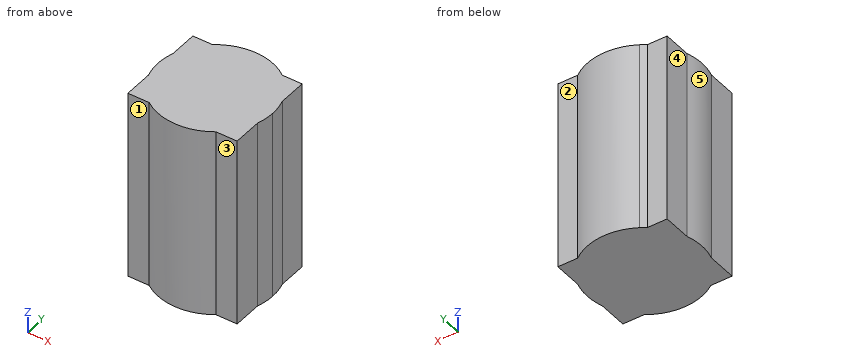
```python
from build123d import *

# Parameters (mm, degrees)
F1_DEPTH = 50.8


with BuildPart() as f1:
    # F0 (on Top) → F1 (new body)
    with BuildSketch(Plane.XY):
        with BuildLine():
            ThreePointArc((14.5472735167, -4.6368075466), (15.087019572, -2.3462718145), (15.2683709345, 0))
            ThreePointArc((15.2683709345, 0), (15.087019572, 2.3462718145), (14.5472735167, 4.6368075466))
            Line((14.5472735167, 4.6368075466), (14.5472735167, -4.6368075466))
        make_face()
        with BuildLine():
            Line((14.5472735167, -4.6368075466), (14.5472735167, 4.6368075466))
            ThreePointArc((14.5472735167, 4.6368075466), (12.4889100158, 8.783523075), (9.2823821573, 12.1227279305))
            Line((9.2823821573, 12.1227279305), (0, 12.1227279305))
            Line((0, 12.1227279305), (-7.8358159836, 12.1227279305))
            Line((-7.8358159836, 12.1227279305), (-9.2823821573, 12.1227279305))
            ThreePointArc((-9.2823821573, 12.1227279305), (-12.4889108979, 8.7835218208), (-14.547274448, 4.6368046247))
            Line((-14.547274448, 4.6368046247), (-14.547274448, -4.6368046247))
            ThreePointArc((-14.547274448, -4.6368046247), (-12.3495786547, -8.9783661121), (-8.8974988368, -12.4079678208))
            Line((-8.8974988368, -12.4079678208), (8.8974988368, -12.4079678208))
            ThreePointArc((8.8974988368, -12.4079678208), (12.349577753, -8.9783673524), (14.5472735167, -4.6368075466))
        make_face()
        with BuildLine():
            ThreePointArc((9.2823821573, 12.1227279305), (12.4889100158, 8.783523075), (14.5472735167, 4.6368075466))
            Line((14.5472735167, 4.6368075466), (14.5472735167, 12.1227279305))
            Line((14.5472735167, 12.1227279305), (9.2823821573, 12.1227279305))
        make_face()
        with BuildLine():
            Line((14.5472735167, -12.4079678208), (14.5472735167, -4.6368075466))
            ThreePointArc((14.5472735167, -4.6368075466), (12.349577753, -8.9783673524), (8.8974988368, -12.4079678208))
            Line((8.8974988368, -12.4079678208), (14.5472735167, -12.4079678208))
        make_face()
        with BuildLine():
            Line((0, 12.1227279305), (9.2823821573, 12.1227279305))
            ThreePointArc((9.2823821573, 12.1227279305), (0.8740812186, 15.2433307717), (-7.8358159836, 13.1043175658))
            Line((-7.8358159836, 13.1043175658), (-7.8358159836, 12.1227279305))
            Line((-7.8358159836, 12.1227279305), (0, 12.1227279305))
        make_face()
        with BuildLine():
            ThreePointArc((-8.8974988368, -12.4079678208), (0, -15.2683709345), (8.8974988368, -12.4079678208))
            Line((8.8974988368, -12.4079678208), (-8.8974988368, -12.4079678208))
        make_face()
        with BuildLine():
            Line((-7.8358159836, 12.1227279305), (-7.8358159836, 13.1043175658))
            ThreePointArc((-7.8358159836, 13.1043175658), (-8.5731590707, 12.6342429351), (-9.2823821573, 12.1227279305))
            Line((-9.2823821573, 12.1227279305), (-7.8358159836, 12.1227279305))
        make_face()
        with BuildLine():
            Line((-14.547274448, -12.4079678208), (-8.8974988368, -12.4079678208))
            ThreePointArc((-8.8974988368, -12.4079678208), (-12.3495786547, -8.9783661121), (-14.547274448, -4.6368046247))
            Line((-14.547274448, -4.6368046247), (-14.547274448, -12.4079678208))
        make_face()
        with BuildLine():
            ThreePointArc((-14.547274448, 4.6368046247), (-12.4889108979, 8.7835218208), (-9.2823821573, 12.1227279305))
            Line((-9.2823821573, 12.1227279305), (-14.547274448, 12.1227279305))
            Line((-14.547274448, 12.1227279305), (-14.547274448, 4.6368046247))
        make_face()
        with BuildLine():
            ThreePointArc((-14.547274448, 4.6368046247), (-15.2683709345, 0), (-14.547274448, -4.6368046247))
            Line((-14.547274448, -4.6368046247), (-14.547274448, 4.6368046247))
        make_face()
    extrude(amount=F1_DEPTH)


solid = f1.part
```
The listing builds one solid part. Answer for the finished solid, in the listing's coordinates (mm). Face numbers are marked on the shaded views. A direction names the side the tool comes from. Give positions to 0.01 mm unless a question says otherwise; leave off trailing zeros. Order: outer loops, then holes, each group sorted by start corner. A loop starts at its lowest first (then second) coordinate and runs counter-clockwise, first axis right, second up. Notation, with made-up numbers: (26, 29) - (31, 29) arc R25 cw to (31, 50) - close; hole circle Ø11 at (60.25, 53.5). An arc over 180 degrees is marked (long way). Answer in a Markdown table with one row per item. Add a question column.
Q1. The part is cut by section C-C (x = 12). Determine the outline of the cut face in (y, z).
Q2. Given P1, Ø8.5, axis at y = -8, z = 17, coming from the -X side; P2, Ø6, axis at x = -11.5, z = 37, coming from the -Y side; P3, Ø6, axis at y = -7.5, z = 27.5, coming from the +X side, each flat-ended and moving along its own axis, determine where each tip first touches the part or whether it passes through.
Q3. The part is cut by section B-B (y = -10.5). Determine the outline of the cut face in (x, z), then the cut area to 3 significant figures.
Q4. Which of the six approach directions +Z, -Z, +X, -X, +Y, -Y give full straight-line access (tool end or side, diameter ignored) to the marked faces 1, 2, 3, 4 and 5?
Q5. Find the intervals of material crossed by line 1 along X through (y, z) = (8, 32); line 2 along Y through (x, z) = (12.5, 38.5); line 3 along Y through (x, z) = (8, 9), in increasing order. Write a range as [from, to].
Q6. The part is cut by section A-A (z = 7). Determine the outline of the cut face in (x, y), then the cut area to 3 significant figures.
Determined:
| question | item | result |
|---|---|---|
| 1 | outline | (-12.41, 0) - (12.12, 0) - (12.12, 50.8) - (-12.41, 50.8) - close |
| 2 | P1 | stops at x = -14.8 |
| 2 | P2 | stops at y = -12.68 |
| 2 | P3 | stops at x = 14.59 |
| 3 | outline | (-14.55, 0) - (14.55, 0) - (14.55, 50.8) - (-14.55, 50.8) - close |
| 3 | area | 1,480 mm² |
| 4 | face 1 | +Z, -Z, -X, -Y |
| 4 | face 2 | +Z, -Z, +X, +Y |
| 4 | face 3 | +Z, -Z, +X, -Y |
| 4 | face 4 | +Z, -Z, -X, +Y |
| 4 | face 5 | +Z, -Z, -X |
| 5 | line 1 | x = [-14.55, 14.55] |
| 5 | line 2 | y = [-12.41, 12.12] |
| 5 | line 3 | y = [-13, 13] |
| 6 | outline | (-14.55, -12.41) - (-8.9, -12.41) arc R15.27 ccw to (8.9, -12.41) - (14.55, -12.41) - (14.55, -4.64) arc R15.27 ccw to (14.55, 4.64) - (14.55, 12.12) - (9.28, 12.12) arc R15.27 ccw to (-9.28, 12.12) - (-14.55, 12.12) - (-14.55, 4.64) arc R15.27 ccw to (-14.55, -4.64) - close |
| 6 | area | 797 mm² |
